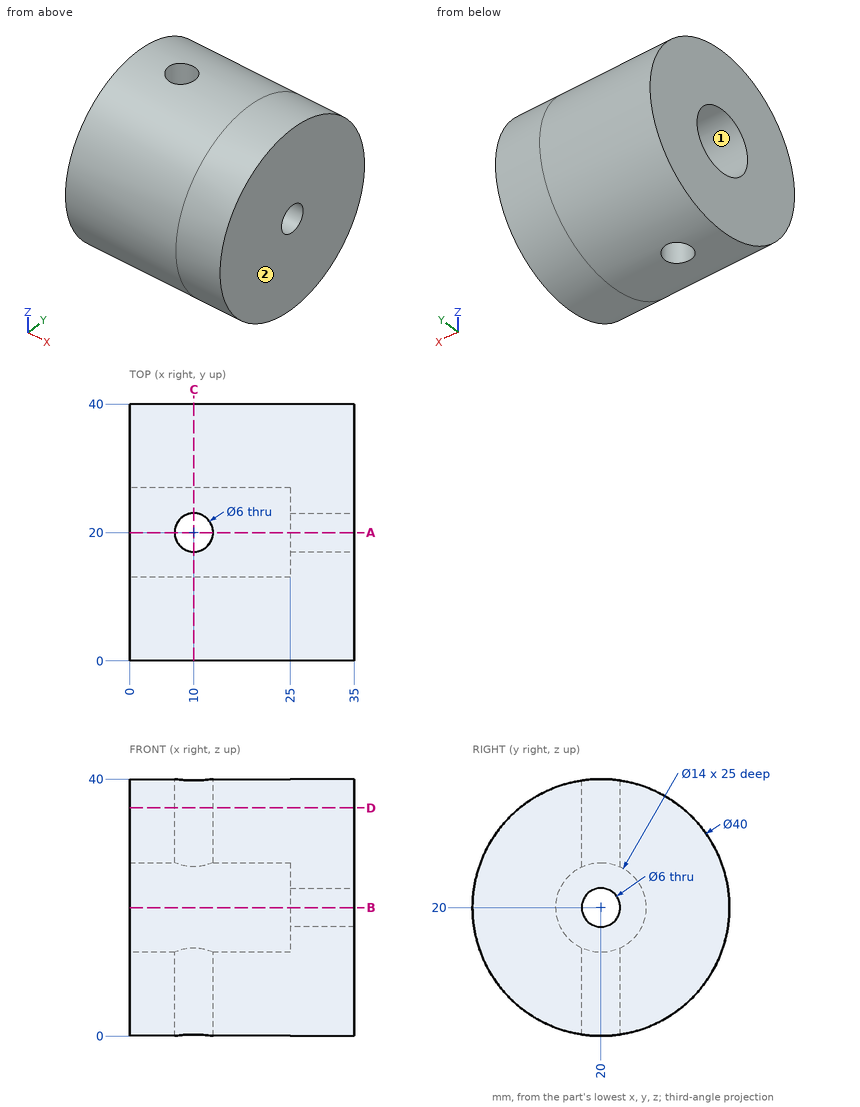
The drawing under review shows one solid part. Ordinate dimensions are in mm from its lowest x, y, z. Round coordinates to 2 decimals unless told otherwise and drop trailing zeros. Order: outer loops, then holes, each group sorted by start corner. A loop starts at its lowest first (then second) coordinate and runs counter-clockwise, first axis right, second up. Notation, with made-up numbers: (14, -3.5) - (61, -3.5) arc R20 ccw to (61, 29.5) - close; hole circle Ø2 at (16, -35). An arc over 180 degrees is marked (long way). Return JSON: item names as keys, results as strings.
Q1. Wall thickness on L1, parallel to Y at x = 16.5, z = 20; L2, parallel to X at y = 15.5, z = 19.5; L3, parallel to Y at x = 9, z = 23: over which ranges is each line inside the solid? List them lowest first. Write a range as [from, to].
Computed values:
{"L1": "y = [0, 13], [27, 40]", "L2": "x = [25, 35]", "L3": "y = [0.23, 13.68], [26.32, 39.77]"}
Q2. The part is to be moulded in two halves that separate along Z. For the marked faces 1 and 2, say which applies: pulls with the +Z half, pulls with the -Z half, needs draft (parallel to the pull), parting line crosses it, or undercut.
Computed values:
{"face 1": "undercut", "face 2": "needs draft"}
Q3. Consider section D-D on z = 35.5. Write out the cut boundary in (x, y), plus the area to 3 significant figures.
Computed values:
{"outline": "(0, 7.36) - (35, 7.36) - (35, 32.64) - (0, 32.64) - close; hole circle Ø6 at (10, 20)", "area": "856 mm2"}
Q4. For pin 1 Ø18 at (y, z) = (20, 20) entering from +X; pin 2 Ø8 at (x, z) = (17.5, 8) entering from +Y; pin 3 Ø5 at (x, z) = (13, 25.5) entering from +Y; pin 4 Ø2 at (x, y) = (12, 24.5) entering from +Z, all flat-tipped, find the tip position at first contact; note any pin that passes through.
Computed values:
{"pin 1": "stops at x = 35", "pin 2": "stops at y = 38.33", "pin 3": "stops at y = 39.77", "pin 4": "stops at z = 39.69"}
Q5. Consider section A-A on y = 20. Write out the cut boundary in (x, z).
Computed values:
{"outline": "(0, 0) - (7, 0) - (7, 13) - (0, 13) - close; (0, 27) - (7, 27) - (7, 40) - (0, 40) - close; (13, 0) - (35, 0) - (35, 17) - (25, 17) - (25, 13) - (13, 13) - close; (13, 27) - (25, 27) - (25, 23) - (35, 23) - (35, 40) - (13, 40) - close"}
Q6. Consider section C-C on x = 10. Write out the cut boundary in (y, z), plus the area to 3 significant figures.
Computed values:
{"outline": "(17, 0.23) - (17, 13.68) arc R7 cw to (17, 26.32) - (17, 39.77) arc R20 ccw to start; (23, 0.23) arc R20 ccw to (23, 39.77) - (23, 26.32) arc R7 cw to (23, 13.68) - close", "area": "945 mm2"}
Q7. Consider section B-B on z = 20. Write out the cut boundary in (x, y), plus the area to 3 significant figures.
Computed values:
{"outline": "(0, 0) - (35, 0) - (35, 17) - (25, 17) - (25, 13) - (0, 13) - close; (0, 27) - (25, 27) - (25, 23) - (35, 23) - (35, 40) - (0, 40) - close", "area": "990 mm2"}
